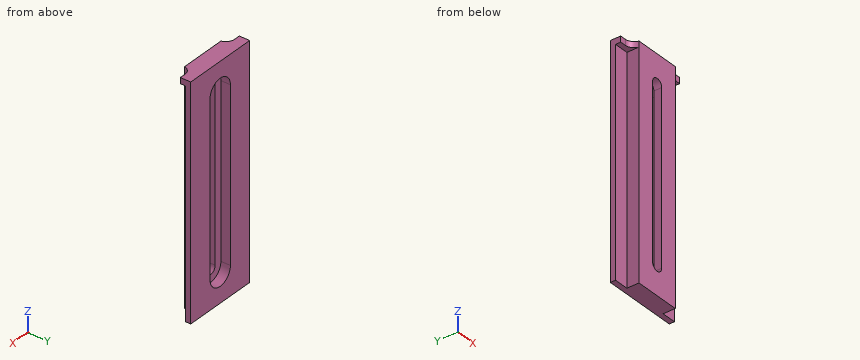
from build123d import *

# Parameters (mm, degrees)
DODANIE_WYCI_GNI_CIE1_DEPTH = 79
WYTNIJ_WYCI_GNI_CIE1_DEPTH  = 81.286985247
WYTNIJ_WYCI_GNI_CIE2_DEPTH  = 3.3
SZKIC5_W                    = 26
SZKIC5_H                    = 3.6
SDF_DEPTH                   = 2
ZAOKR_GLENIE3_R             = 3


with BuildPart() as part:
    # Szkic1 → Dodanie-wyciągnięcie1 (new body)
    with BuildSketch(Plane.XY):
        Polygon((-13, 0), (-13, 1.8), (13, 1.8), (13, 0), (8, 0), (8, -4.2), (-8, -4.2), (-8, 0), align=None)
    extrude(amount=DODANIE_WYCI_GNI_CIE1_DEPTH)

    # Szkic3 → Wytnij-wyciągnięcie1 (cut, through all)
    with BuildSketch(Plane.XZ.offset(4.2)):
        with BuildLine():
            Line((2, 69), (2, 10))
            ThreePointArc((2, 10), (0, 8), (-2, 10))
            Line((-2, 10), (-2, 69))
            ThreePointArc((-2, 69), (0, 71), (2, 69))
        make_face()
    extrude(amount=-WYTNIJ_WYCI_GNI_CIE1_DEPTH, mode=Mode.SUBTRACT)

    # Szkic4 → Wytnij-wyciągnięcie2 (cut)
    with BuildSketch(Plane(origin=(0, 1.8, 0), x_dir=(1, 0, 0), z_dir=(0, 1, 0))):
        with BuildLine():
            Line((-4.5, -69), (-4.5, -10))
            ThreePointArc((-4.5, -10), (0, -5.5), (4.5, -10))
            Line((4.5, -10), (4.5, -69))
            ThreePointArc((4.5, -69), (0, -73.5), (-4.5, -69))
        make_face()
    extrude(amount=-WYTNIJ_WYCI_GNI_CIE2_DEPTH, mode=Mode.SUBTRACT)

    # Szkic5 → sdf (add)
    with BuildSketch(Plane.XY.offset(79)):
        Rectangle(SZKIC5_W, SZKIC5_H)
    extrude(amount=-SDF_DEPTH)

    # Zaokrąglenie3
    # the kernel refuses this fillet: 3 mm, written as the material it adds along each edge
    with BuildSketch(Plane(origin=(8, -1.8, 77), x_dir=(1.5609735726224723e-12, -1.0, 0), z_dir=(0, 0, 1)), Plane(origin=(-8, -1.8, 79), x_dir=(-1.5698553568194677e-12, -1.0, 0), z_dir=(0, 0, -1))) as zaokr_glenie3_piece_1:
        with BuildLine():
            CenterArc((3, 2.939387691), ZAOKR_GLENIE3_R, 180, 78.463040967)
            Line((0, 2.939387691), (-0.06, 2.939387691))
            Line((-0.06, 2.939387691), (-0.06, 0))
            Line((-0.06, 0), (0, -0.06))
            ThreePointArc((0, -0.06), (1.2, -0.06), (2.388, -0.058787754))
            Line((2.388, -0.058787754), (2.4, 0))
        make_face()
    extrude(amount=2)


solid = part.part
Verification items for the finished model (mm, model axes). Coordinates: 2 decimals unless noted, no trailing zeros. Order: outer loops, then holes, each group sorted by start corner. A loop starts at its lowest first (then second) coordinate and runs counter-clockwise, first axis right, second up. Notation, with made-up numbers: (56, 7.5) -> (115, 7.5) arc R14 ccw to (115, 19.5) -> close; hole circle Ø4 at (-11, 47.5). An arc over 180 degrees is marked (long way). Put each result on its own line as item: value. Start each with the question number.
1. Material ranges on L1, parallel to X at y = -1.05, z = 65; L2, parallel to X at y = -1.8, z = 51; L3, parallel to Y at x = 3.25, z = 7, recorded low to high. Write a range as [from, to].
2. Cross-section at B-B, the plane x = 0. Record the boundary of the cut face in (y, z).
3. Go/stop test with flat-tipped pins: pin 1 Ø2 at (x, y) = (9.5, -2.5) entering from -Z; pin 2 Ø1.5 at (x, y) = (-0.5, -2) entering from -Z; pin 3 Ø1 at (x, z) = (12.5, 77.5) entering from -Y; pin 4 Ø4 at (x, z) = (1, 59) entering from +Y. Record where each tip stops, or that it passes through.
4. Cross-section at A-A, the plane z = 55. Record the boundary of the cut face in (x, y).
Computed:
1. L1: [-8, -4.5], [4.5, 8]
1. L2: [-8, -2], [2, 8]
1. L3: [-4.2, -1.5]
2. outline: (-4.2, 0) -> (1.8, 0) -> (1.8, 5.5) -> (-1.5, 5.5) -> (-1.5, 8) -> (-4.2, 8) -> close; (-4.2, 71) -> (-1.5, 71) -> (-1.5, 73.5) -> (1.8, 73.5) -> (1.8, 79) -> (-4.2, 79) -> close
3. pin 1: z = 77
3. pin 2: z = 0
3. pin 3: y = -1.8
3. pin 4: y = -1.5
4. outline: (-13, 0) -> (-8, 0) -> (-8, -4.2) -> (-2, -4.2) -> (-2, -1.5) -> (-4.5, -1.5) -> (-4.5, 1.8) -> (-13, 1.8) -> close; (2, -4.2) -> (8, -4.2) -> (8, 0) -> (13, 0) -> (13, 1.8) -> (4.5, 1.8) -> (4.5, -1.5) -> (2, -1.5) -> close
